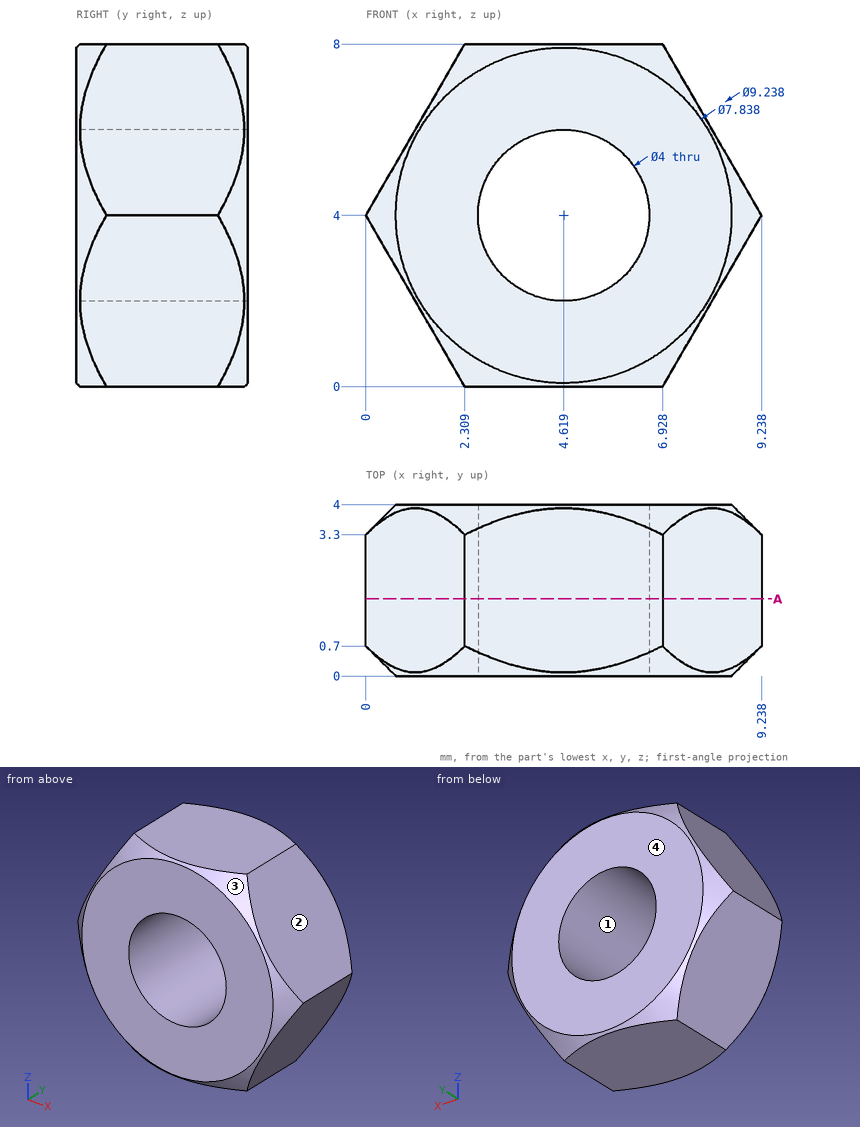
The drawing under review shows one solid part. Ordinate dimensions are in mm from its lowest x, y, z. Round coordinates to 2 decimals unless told otherwise and drop trailing zeros. Write each loop counter-clockwise with the first axis right and the second up, starting at its lowest first coordinate (ties: lowest second). Pieces come first, ordered by that corner, then holes.
(1) Wall thickness on L1, parallel to X at y = 3.1, z = 5.25 (1 decimal); L2, parallel to X at y = 3.3, z = 3.25 (1 decimal); L3, parallel to Z at x = 4.5, y = 3.4: over which ranges is each line inside the solid? List them lowest first.
(2) We need section A-A on y = 1.8. Give the boundary of the cut face in (x, z).
(3) Insertion check: pin 1 (1 mm diameter, centred on x = 1.5, y = 1, fed in from -Z) (1 decimal). The pin has a flat end and moves straight along its axis. Give the tip position at first contact, or say it passes through.
(4) Mouldability with a two-part tool opening along X and no side actions: class the marked faces 1, 2, 3 and 4 as +X half, -X half, draft (parallel to the pull), parting line (faces both ways), or undercut.
Findings below:
1. L1: x = 0.7 to 3.1, 6.2 to 8.5
1. L2: x = 0.4 to 2.8, 6.5 to 8.8
1. L3: z = 0 to 2, 6 to 8
2. outline: (0, 4) - (2.31, 0) - (6.93, 0) - (9.24, 4) - (6.93, 8) - (2.31, 8) - close; hole circle Ø4 at (4.62, 4)
3. pin 1: stops at z = 0.5
4. face 1: undercut
4. face 2: +X half
4. face 3: parting line
4. face 4: draft
